from build123d import *

# Parameters (mm, degrees)
BOSS_EXTRUDE4_DEPTH = 32.4358
SKETCH4_R           = 10.9982
BOSS_EXTRUDE5_DEPTH = 2.54
SKETCH5_R           = 2.4892
BOSS_EXTRUDE6_DEPTH = 11.3284
SKETCH6_R           = 1.3716
BOSS_EXTRUDE7_DEPTH = 6.35
BOSS_EXTRUDE8_START = 0.9144
SKETCH7_R           = 2.4892
BOSS_EXTRUDE8_DEPTH = 0.9144


with BuildPart() as part:
    # Sketch1 → Boss-Extrude4 (new body)
    with BuildSketch(Plane.XY):
        Polygon((0, 4.077036279), (4.077036279, 0), (37.959963721, 0), (42.037, 4.077036279), (42.037, 38.086963721), (37.959963721, 42.164), (4.070882272, 42.164), (0, 38.08081899), align=None)
    extrude(amount=BOSS_EXTRUDE4_DEPTH)

    # Sketch4 → Boss-Extrude5 (add)
    with BuildSketch(Plane.XY.offset(32.4358)):
        with Locations((21.0185, 21.078927634)):
            Circle(SKETCH4_R)
    extrude(amount=BOSS_EXTRUDE5_DEPTH)

    # Sketch5 → Boss-Extrude6 (add)
    with BuildSketch(Plane.XY.offset(34.9758)):
        with Locations(Location((21.0185, 21.078927634, 0), (0, 0, 180))):
            Circle(SKETCH5_R)
    extrude(amount=BOSS_EXTRUDE6_DEPTH)

    # Sketch6 → Boss-Extrude7 (add)
    with BuildSketch(Plane.XY.offset(32.4358)):
        with Locations((4.826, 37.338)):
            Circle(SKETCH6_R)
        with Locations((4.826, 4.826)):
            Circle(SKETCH6_R)
        with Locations((37.211, 4.826)):
            Circle(SKETCH6_R)
        with Locations((37.211, 37.338)):
            Circle(SKETCH6_R)
    extrude(amount=BOSS_EXTRUDE7_DEPTH)

    # Sketch7 → Boss-Extrude8 (add)
    with BuildSketch(Plane(origin=(0, 0, 0), x_dir=(-1, 0, 0), z_dir=(0, 0, -1)).offset(BOSS_EXTRUDE8_START)):
        with Locations((-21.0185, 21.078927634)):
            Circle(SKETCH7_R)
    extrude(amount=-BOSS_EXTRUDE8_DEPTH)


solid = part.part
Geometry: final body of the model. Coordinates: model frame, mm. A direction names the side the tool comes from. Coordinates: 2 decimals unless noted, no trailing zeros. Write each loop counter-clockwise with the first axis right and the second up, starting at its lowest first coordinate (ties: lowest second). Pieces come first, ordered by that corner, then holes. Notation, with made-up numbers: (46.5, 21.25) - (60.5, 21.25) arc R11 cw to (60.5, 36.25) - close; hole circle Ø10 at (31.25, -1.5). An arc over 180 degrees is marked (long way). Return JSON: item names as keys, results as strings.
Item 1: Section query B-B (y = 29). Output: boundary loops of the cut face in (x, z), and give its area (3 significant figures).
Completed:
{"outline": "(0, 0) - (42.04, 0) - (42.04, 32.44) - (28.65, 32.44) - (28.65, 34.98) - (13.39, 34.98) - (13.39, 32.44) - (0, 32.44) - close", "area": "1,400 mm2"}
Item 2: Pin query (flat end, axial travel): pin 1 Ø0.8 at (x, y) = (4.5, 4.5) entering from +Z; pin 2 Ø10 at (x, y) = (32, 27) entering from +Z; pin 3 Ø1.5 at (x, y) = (33, 20) entering from +Z. Return the tip coordinate at first contact, or that it passes through.
Completed:
{"pin 1": "stops at z = 38.79", "pin 2": "stops at z = 34.98", "pin 3": "stops at z = 32.44"}
Item 3: Section query A-A (z = 16). Output: boundary loops of the cut face in (x, y).
Completed:
{"outline": "(0, 4.08) - (4.08, 0) - (37.96, 0) - (42.04, 4.08) - (42.04, 38.09) - (37.96, 42.16) - (4.07, 42.16) - (0, 38.08) - close"}
Item 4: Section query D-D (x = 33.5). Output: boundary loops of the cut face in (y, z).
Completed:
{"outline": "(0, 0) - (42.16, 0) - (42.16, 32.44) - (0, 32.44) - close"}
Item 5: Section query C-C (x = 22). Output: boundary loops of the cut face in (y, z).
Completed:
{"outline": "(0, 0) - (18.79, 0) - (18.79, -0.91) - (23.37, -0.91) - (23.37, 0) - (42.16, 0) - (42.16, 32.44) - (32.03, 32.44) - (32.03, 34.98) - (23.37, 34.98) - (23.37, 46.3) - (18.79, 46.3) - (18.79, 34.98) - (10.12, 34.98) - (10.12, 32.44) - (0, 32.44) - close"}
Item 6: Line query: L1, parallel to Z at x = 28, y = 29; L2, parallel to Z at x = 8, y = 16; L3, parallel to X at y = 4, z = 35.5. Output: solid intervals per line, ascending.
Completed:
{"L1": "z = 0 to 34.98", "L2": "z = 0 to 32.44", "L3": "x = 3.73 to 5.92, 36.12 to 38.31"}
Item 7: Pull-direction query (Y, two-part tool) for faces 3 (the face through (38.52, 5.24, 35.57)), 4 (the face through (18.719, 20.126, -0.464)), 5 (the face through (21, 42.164, 16)), 6 (the face through (21, 24, 34.976)); classes: +Y half, -Y half, draft (parallel to the pull), parting line (faces both ways), or undercut.
Completed:
{"face 3": "undercut", "face 4": "parting line", "face 5": "+Y half", "face 6": "draft"}
Item 8: Reachability of faces 1 (the face through (30, 12, 32.436)), 2 (the face through (39.97, 2.01, 15.99)) from +Z, -Z, +X, -X, +Y, -Y: full face, straight path, thin tool, end or side. Return the list, or none.
Completed:
{"face 1": "+Z", "face 2": "+Z, -Z, +X, -Y"}
